Input: part model. Units: mm. Frame: model coordinates. A direction names the side the tool comes from. Give positions to 0.01 mm unless a question says otherwise; leave off trailing zeros. Loops run counter-clockwise (first coordinate to the right, second up) from the corner with the lowest first, then second, coordinate; pieces in that order, holes last. Notation, with made-up numbers: (-24.5, 4) - (-2.5, 4) arc R20 cw to (-2.5, 16) - close; hole circle Ø4 at (42.5, 85). An arc over 180 degrees is marked (long way). One line per question, with ' | ' between items. Start each with the question number.
from build123d import *

# Parameters (mm, degrees)
ESBO_O1_W                                      = 85
ESBO_O1_H                                      = 45
RESSALTO_EXTRUS_O1_DEPTH                       = 35
ESBO_O2_W                                      = 81
ESBO_O2_H                                      = 41
CORTE_EXTRUS_O1_DEPTH                          = 33
ESBO_O3_W                                      = 2
ESBO_O3_H                                      = 45
RESSALTO_EXTRUS_O2_DEPTH                       = 15
RESSALTO_EXTRUS_O3_DEPTH                       = 15
ESBO_O5_W                                      = 2
ESBO_O5_H                                      = 45
RESSALTO_EXTRUS_O4_DEPTH                       = 15
ESBO_O6_W                                      = 85
ESBO_O6_H                                      = 2
RESSALTO_EXTRUS_O5_DEPTH                       = 15
BROCA_DE_ROSQUEAR_DE_CANO_PARA_TARRAXA_D_D     = 6.579997
BROCA_DE_ROSQUEAR_DE_CANO_PARA_TARRAXA_D_DEPTH = 10
BROCA_DE_ROSQUEAR_DE_CANO_PARA_TARRAXA_D_TIP   = 1.976830535
CORTE_EXTRUS_O2_REACH                          = 37
ESBO_O9_W                                      = 81
ESBO_O9_H                                      = 41


with BuildPart() as part:
    # Esboço1 → Ressalto-extrusão1 (new body)
    with BuildSketch(Plane.XY):
        Rectangle(ESBO_O1_W, ESBO_O1_H)
    extrude(amount=RESSALTO_EXTRUS_O1_DEPTH)

    # Esboço2 → Corte-extrusão1 (cut)
    with BuildSketch(Plane(origin=(0, 0, 0), x_dir=(-1, 0, 0), z_dir=(0, 0, -1))):
        Rectangle(ESBO_O2_W, ESBO_O2_H)
    extrude(amount=-CORTE_EXTRUS_O1_DEPTH, mode=Mode.SUBTRACT)

    # Esboço3 → Ressalto-extrusão2 (add)
    with BuildSketch(Plane(origin=(42.5, 0, 0), x_dir=(0, 0, -1), z_dir=(1, 0, 0))):
        with Locations((-1, 0)):
            Rectangle(ESBO_O3_W, ESBO_O3_H)
    extrude(amount=RESSALTO_EXTRUS_O2_DEPTH)

    # Esboço4 → Ressalto-extrusão3 (add)
    with BuildSketch(Plane(origin=(0, 22.5, 0), x_dir=(1, 0, 0), z_dir=(0, 1, 0))):
        Polygon((42.397707887, 0), (42.5, -2), (-42.5, -2), (-42.5, 0), align=None)
    extrude(amount=RESSALTO_EXTRUS_O3_DEPTH)

    # Esboço5 → Ressalto-extrusão4 (add)
    with BuildSketch(Plane.ZY.offset(42.5)):
        with Locations((1, 0)):
            Rectangle(ESBO_O5_W, ESBO_O5_H)
    extrude(amount=RESSALTO_EXTRUS_O4_DEPTH)

    # Esboço6 → Ressalto-extrusão5 (add)
    with BuildSketch(Plane.XZ.offset(22.5)):
        with Locations((0, 1)):
            Rectangle(ESBO_O6_W, ESBO_O6_H)
    extrude(amount=RESSALTO_EXTRUS_O5_DEPTH)

    # Broca de rosquear de cano para tarraxa de 1/81
    with Locations(Plane.XY.offset(2)):
        with Locations((50, 11.25), (50, -11.25), (-51.152400613, -11.25), (-51.152400613, 11.25), (-28.33, 30), (0, 30), (28.33, 30), (28.33, -30), (0, -30), (-28.33, -30)):
            Hole(BROCA_DE_ROSQUEAR_DE_CANO_PARA_TARRAXA_D_D / 2, depth=BROCA_DE_ROSQUEAR_DE_CANO_PARA_TARRAXA_D_DEPTH)
            with Locations((0, 0, -(BROCA_DE_ROSQUEAR_DE_CANO_PARA_TARRAXA_D_DEPTH + BROCA_DE_ROSQUEAR_DE_CANO_PARA_TARRAXA_D_TIP / 2))):  # 118° drill point
                Cone(0, BROCA_DE_ROSQUEAR_DE_CANO_PARA_TARRAXA_D_D / 2, BROCA_DE_ROSQUEAR_DE_CANO_PARA_TARRAXA_D_TIP, mode=Mode.SUBTRACT)

    # Esboço9 → Corte-extrusão2 (cut, up to next)
    with BuildSketch(Plane.XY.offset(35), mode=Mode.PRIVATE) as corte_extrus_o2_sk1:
        Rectangle(ESBO_O9_W, ESBO_O9_H)
    corte_extrus_o2_tool1 = extrude(corte_extrus_o2_sk1.sketch, amount=-CORTE_EXTRUS_O2_REACH, mode=Mode.PRIVATE) & part.part
    add(corte_extrus_o2_tool1.solids().sort_by_distance((0, 0, 35))[0], mode=Mode.SUBTRACT)


solid = part.part
Q1. Line query: L1, parallel to Y at x = 0, z = 1.15; L2, parallel to Y at x = -22, z = 22; L3, parallel to X at y = -2.5, z = 17.5. Output: solid intervals per line, ascending. Write a range as from..to.
Q2. Access query for faces 1 (the face through (1, -20.5, 17)), 2 (the face through (42.5, 0, 18)), 3 (the face through (-1, 26, 0)), 4 (the face through (-1, 22.5, 19)), 5 (the face through (-3, -22, 35)). Directions: +Z, -Z, +X, -X, +Y, -Y. A direction counts if a zero-diameter tool reaches every point of the face in a straight line with its end or side. Return the directions, or none.
Q3. Draft query along Y for faces 6 (the face through (1, -22.5, 18)), 7 (the face through (-0.6, -26.6, 2)), 8 (the face through (30.755, -27.776, 0.986)), 9 (the face through (30.755, 32.224, 0.986)). Return one class per face: +Y half, -Y half, draft (parallel to the pull), parting line (faces both ways), or undercut.
Q4. First-contact query: pin 1 (4.5 mm diameter, centred on x = 14.5, y = 32, fed in from +Z); pin 2 (3 mm diameter, centred on x = -39.5, y = -6, fed in from -Z); pin 3 (4 mm diameter, centred on y = -3, z = 27, fed in from +X); pin 4 (6 mm diameter, centred on x = 10.5, z = 27, fed in from -Y). Flat tips, straight axial feed; report the tip coordinate or a pass-through.
Q5. Section C-C, the plane x = 50. Output: boundary loops of the cut face in (y, z), plus the area to 3 significant figures.
Q6. Section D-D, the plane z = 12.5. Output: boundary loops of the cut face in (x, y), plus the area to 3 significant figures.
Q7. Section B-B, the plane y = 11.25. Output: boundary loops of the cut face in (x, z), plus the area to 3 significant figures.
Q8. Section A-A, the plane x = -28.33. Output: boundary loops of the cut face in (y, z), plus the area to 3 significant figures.
Solved:
1) L1: y = -37.5..-33.29, -26.71..-20.5, 20.5..26.71, 33.29..37.5 | L2: y = -22.5..-20.5, 20.5..22.5 | L3: x = -42.5..-40.5, 40.5..42.5
2) face 1: +Z, -Z | face 2: +Z, +X, +Y, -Y | face 3: -Z, +X, -X, +Y, -Y | face 4: +Z, +X, -X, +Y | face 5: +Z, +X, -X, +Y, -Y
3) face 6: -Y half | face 7: draft | face 8: undercut | face 9: undercut
4) pin 1: stops at z = 2 | pin 2: stops at z = 0 | pin 3: stops at x = 42.5 | pin 4: stops at y = -22.5
5) outline: (-22.5, 0) - (-14.54, 0) - (-14.54, 2) - (-22.5, 2) - close; (-7.96, 0) - (7.96, 0) - (7.96, 2) - (-7.96, 2) - close; (14.54, 0) - (22.5, 0) - (22.5, 2) - (14.54, 2) - close | area: 63.7 mm²
6) outline: (-42.5, -22.5) - (42.5, -22.5) - (42.5, 22.5) - (-42.5, 22.5) - close; hole (-40.5, -20.5) - (40.5, -20.5) - (40.5, 20.5) - (-40.5, 20.5) - close | area: 504 mm²
7) outline: (-57.5, 0) - (-54.44, 0) - (-54.44, 2) - (-57.5, 2) - close; (-47.86, 0) - (-40.5, 0) - (-40.5, 35) - (-42.5, 35) - (-42.5, 2) - (-47.86, 2) - close; (40.5, 0) - (46.71, 0) - (46.71, 2) - (42.5, 2) - (42.5, 35) - (40.5, 35) - close; (53.29, 0) - (57.5, 0) - (57.5, 2) - (53.29, 2) - close | area: 174 mm²
8) outline: (-37.5, 0) - (-33.29, 0) - (-33.29, 2) - (-37.5, 2) - close; (-26.71, 0) - (-20.5, 0) - (-20.5, 35) - (-22.5, 35) - (-22.5, 2) - (-26.71, 2) - close; (20.5, 0) - (26.71, 0) - (26.71, 2) - (22.5, 2) - (22.5, 35) - (20.5, 35) - close; (33.29, 0) - (37.5, 0) - (37.5, 2) - (33.29, 2) - close | area: 174 mm²
